CAD build for the part. Positions are in the model's coordinates, mm. A direction names the side the tool comes from. Give positions to 0.01 mm unless a question says otherwise; leave off trailing zeros. Order: outer loops, then holes, each group sorted by start corner. A loop starts at its lowest first (then second) coordinate and runs counter-clockwise, first axis right, second up.
Item 1: Wall check: L1, parallel to Z at x = -55, y = 7; L2, parallel to Z at x = -55, y = 10.25; L3, parallel to X at y = 7.25, z = 16. Give the ranges that are in metal, low to high.
Item 2: Band-saw the part on A-A on x = -55. Give the cut face in (y, z).
Item 3: Two-plate mould, pull along Z, no slides. Class faces 1 (the flat face through (-67.5, 5, 8)), 2 (the cylindrical face through (-55, 7, 53)), 3 (the flat face through (-80.761, 7.395, 39.675)): released by +Z, released by -Z, zero draft, split by the parting line, or undercut.
Item 4: Band-saw the part on D-D on x = -66. Give the cut face in (y, z).
Item 5: Flat gauge pins, fed straight in: P1, Ø6.5, axis at x = -55, z = 55, coming from the +Y side; P2, Ø5, axis at y = 13, z = 41.5, coming from the +X side; P3, Ø4, axis at x = -34.5, z = 46.5, coming from the +Y side; P4, Ø4, axis at y = 12, z = 35.5, coming from the -X side. Where does each tip first touch, or does it go through?
Item 6: Band-saw the part on B-B on y = 4.75. Give the cut face in (x, z).
Item 7: Which spindle directions (+Z, -Z, +X, -X, +Y, -Y) get a long thin tool onto all of the face, cutting with end or side? Do faces 4 (the flat face through (-42.5, 5, 8)), 5 (the flat face through (-29.812, 7.395, 40.098)). Say none if no direction does.
Item 8: Band-saw the part on C-C on z = 19.5. Give the cut face in (x, y), plus the area to 3 significant figures.
Autodesk Inventor part; units mm, degrees
ref_plane "YZ Plane" through (0, 0, 0) normal (1, 0, 0) x (0, 1, 0)
ref_plane "XZ Plane" through (0, 0, 0) normal (0, 1, 0) x (-1, 0, 0)
ref_plane "XY Plane" through (0, 0, 0) normal (0, 0, 1) x (1, 0, 0)
sketch "スケッチ1" plane through (0, 0, 0) normal (0, 1, 0) x (-1, 0, 0)
  arc A0 (9.0513, 24.7723) -> (100.9487, 24.7723) centre (55, 55) ccw
  circle A1 centre (55, 15) radius 12.5
  arc A2 (60, 55) -> (50, 55) centre (55, 55) ccw
  circle A3 centre (55, 55) radius 2
  arc A4 (9.0513, 24.7723) -> (100.9487, 24.7723) centre (55, 55) ccw
  line L0 (100.9487, 24.7723) -> (60, 55)
  line L1 (50, 55) -> (9.0513, 24.7723)
  circle A5 centre (55, 55) radius 5
  arc A6 (60, 55) -> (50, 55) centre (55, 55) ccw
  point P0 (0, 0)
extrude "押し出し1" add sketch "スケッチ1" along normal blind 15
sketch "スケッチ2" plane through (0, 15, 0) normal (0, 1, 0) x (1, 0, 0)
  circle A0 centre (-55, -15) radius 12.5
  circle A1 centre (-55, -15) radius 12.5
  point P0 (0, 0)
extrude "押し出し2" add sketch "スケッチ2" against normal blind 5
sketch "スケッチ3" plane through (0, 0, 0) normal (0, -1, 0) x (1, 0, 0)
  circle A0 centre (-55, 15) radius 12.5
  line L0 (-67.5, 15) -> (-42.5, 15)
  line L1 (-42.5, 15) -> (-42.5, -1.7653)
  line L2 (-42.5, -1.7653) -> (-67.5, -1.7653)
  line L3 (-67.5, -1.7653) -> (-67.5, 15)
  point P0 (0, 0)
extrude "押し出し3" cut sketch "スケッチ3" against normal blind 10 contours L1 L2 L3 A0 | A0 L0 picked at (-57.3669, 11.5709)
properties part number "R_kit_test"
The answers:
1. L1: z = 27.5 to 53, 57 to 60
1. L2: z = 0 to 53, 57 to 60
1. L3: x = -93.78 to -67.46, -42.54 to -16.22
2. outline: (0, 27.5) - (10, 27.5) - (10, 0) - (15, 0) - (15, 53) - (0, 53) - close; (0, 57) - (15, 57) - (15, 60) - (0, 60) - close
3. face 1: zero draft
3. face 2: undercut
3. face 3: released by +Z
4. outline: (0, 20.94) - (10, 20.94) - (10, 1.11) - (15, 1.11) - (15, 50.57) - (0, 50.57) - close
5. P1: stops at y = 15
5. P2: stops at x = -28.33
5. P3: passes through
5. P4: stops at x = -89.13
6. outline: (-100.95, 24.77) arc R55 ccw to (-67.5, 1.44) - (-67.5, 15) arc R12.5 cw to (-42.5, 15) - (-42.5, 1.44) arc R55 ccw to (-9.05, 24.77) - (-50, 55) arc R5 ccw to (-60, 55) - close; hole circle Ø4 at (-55, 55)
7. face 4: -Z, -Y
7. face 5: +Z, +X, +Y, -Y
8. outline: (-97.01, 0) - (-66.66, 0) - (-66.66, 10) - (-43.34, 10) - (-43.34, 0) - (-12.99, 0) - (-12.99, 15) - (-97.01, 15) - close
8. area: 1,030 mm2
